Read the model definition and answer for the solid it produces. Units are mm, in the model's axes. A direction names the side the tool comes from. Give positions to 0.01 mm unless a question says otherwise; leave off trailing zeros. Loops run counter-clockwise (first coordinate to the right, second up) from the corner with the lowest first, then second, coordinate; pieces in that order, holes last. Notation, with made-up numbers: (-35, 46) -> (-29, 46) arc R11 cw to (-29, 51) -> close; hole circle Ø9 at (57.25, -1). An arc over 180 degrees is marked (long way). Return JSON: item names as keys, results as strings. Group by question number.
from build123d import *

# Parameters (mm, degrees)
SKETCH1_W           = 195
SKETCH1_H           = 40
BOSS_EXTRUDE1_DEPTH = 10
SKETCH2_W           = 145
SKETCH2_H           = 40
BOSS_EXTRUDE2_DEPTH = 55
CUT_EXTRUDE1_DEPTH  = 237
FILLET1_R           = 7
CUT_EXTRUDE2_DEPTH  = 237
CUT_EXTRUDE3_DEPTH  = 237
SKETCH6_R           = 3
CUT_EXTRUDE4_DEPTH  = 237
SKETCH7_R           = 17.5
BOSS_EXTRUDE3_DEPTH = 2
BOSS_EXTRUDE4_DEPTH = 6
SKETCH9_R           = 4.5
BOSS_EXTRUDE5_DEPTH = 10
BOSS_EXTRUDE7_DEPTH = 5


with BuildPart() as part:
    # Sketch1 → Boss-Extrude1 (new body)
    with BuildSketch(Plane(origin=(0, 0, 0), x_dir=(1, 0, 0), z_dir=(0, 1, 0))):
        Rectangle(SKETCH1_W, SKETCH1_H)
    extrude(amount=BOSS_EXTRUDE1_DEPTH)

    # Sketch2 → Boss-Extrude2 (add)
    with BuildSketch(Plane(origin=(0, 10, 0), x_dir=(1, 0, 0), z_dir=(0, 1, 0))):
        Rectangle(SKETCH2_W, SKETCH2_H)
    extrude(amount=BOSS_EXTRUDE2_DEPTH)

    # Sketch3 → Cut-Extrude1 (cut)
    with BuildSketch(Plane.ZY.offset(72.5)):
        Polygon((-11.5, 65), (-20, 55), (-20, 68.642587118), align=None)
        Polygon((11.5, 65), (20, 55), (20, 68.642587118), align=None)
    extrude(amount=-CUT_EXTRUDE1_DEPTH, mode=Mode.SUBTRACT)

    # Fillet1
    fillet1_edges = [part.edges().sort_by_distance(p)[0] for p in [
        (0, 55, -20),
        (0, 55, 20),
    ]]
    fillet(fillet1_edges, radius=FILLET1_R)

    # Sketch4 → Cut-Extrude2 (cut)
    with BuildSketch(Plane(origin=(0, 0, -20), x_dir=(-1, 0, 0), z_dir=(0, 0, -1))):
        Polygon((72.5, 10), (97.5, 8), (97.5, 10), align=None)
        Polygon((-97.5, 10), (-72.5, 10), (-97.5, 8), align=None)
    extrude(amount=-CUT_EXTRUDE2_DEPTH, mode=Mode.SUBTRACT)

    # Sketch5 → Cut-Extrude3 (cut)
    with BuildSketch(Plane.XZ):
        Polygon((97.5, -20), (97.5, -17.5), (72.5, -20), align=None)
        Polygon((97.5, 20), (72.5, 20), (97.5, 17.5), align=None)
        Polygon((-97.5, 17.5), (-72.5, 20), (-97.5, 20), align=None)
        Polygon((-72.5, -20), (-97.5, -17.5), (-97.5, -20), align=None)
    extrude(amount=-CUT_EXTRUDE3_DEPTH, mode=Mode.SUBTRACT)

    # Sketch6 → Cut-Extrude4 (cut)
    with BuildSketch(Plane.XZ):
        with Locations((89.5, 9)):
            Circle(SKETCH6_R)
        with Locations((89.5, -9)):
            Circle(SKETCH6_R)
        with Locations((-89.5, 9)):
            Circle(SKETCH6_R)
        with Locations((-89.5, -9)):
            Circle(SKETCH6_R)
    extrude(amount=-CUT_EXTRUDE4_DEPTH, mode=Mode.SUBTRACT)

    # Sketch7 → Boss-Extrude3 (add)
    with BuildSketch(Plane(origin=(0, 0, -20), x_dir=(-1, 0, 0), z_dir=(0, 0, -1))):
        with Locations((0, 22.5)):
            Circle(SKETCH7_R)
    extrude(amount=BOSS_EXTRUDE3_DEPTH)

    # Sketch8 → Boss-Extrude4 (add)
    with BuildSketch(Plane(origin=(0, 0, -22), x_dir=(-1, 0, 0), z_dir=(0, 0, -1))):
        Polygon((8.082903769, 8.5), (16.165807537, 22.5), (8.082903769, 36.5), (-8.082903769, 36.5), (-16.165807537, 22.5), (-8.082903769, 8.5), align=None)
    extrude(amount=BOSS_EXTRUDE4_DEPTH)

    # Sketch9 → Boss-Extrude5 (add)
    with BuildSketch(Plane(origin=(0, 0, -28), x_dir=(-1, 0, 0), z_dir=(0, 0, -1))):
        with Locations((0, 22.5)):
            Circle(SKETCH9_R)
    extrude(amount=BOSS_EXTRUDE5_DEPTH)

    # Sketch12 → Boss-Extrude7 (add)
    with BuildSketch(Plane(origin=(0, 0, -38), x_dir=(-1, 0, 0), z_dir=(0, 0, -1))):
        Polygon((2.100473826, 16.281199441), (6.435876178, 21.209663414), (4.335402352, 27.428463972), (-2.100473826, 28.718800559), (-6.435876178, 23.790336586), (-4.335402352, 17.571536028), align=None)
    extrude(amount=BOSS_EXTRUDE7_DEPTH)


solid = part.part
1. Section D-D on y = 34.5 is taken. Determine the outline of the cut face in (x, z), then the cut area to 3 significant figures.
2. Straight lines are drawn through the part: line 1 (X direction, y = 4, z = -9); line 2 (Z direction, x = 89.5, y = 4); line 3 (Z direction, x = -89, y = 3). For each, find the intervals that lie inside material, in ascending order. Write a range as from..to.
3. Section C-C on z = 0 is taken. Determine the outline of the cut face in (x, y).
4. Determine the mould class of faces 1 (the flat face through (72.5, 37, 0)), 2 (the flat face through (-2, 27, -38)), 3 (the cylindrical face through (86.5, 4.4, 9.1)), 4 (the cylindrical face through (-92.5, 4.4, 9.1)) for opening direction X: pulls with the +X half, pulls with the -X half, needs draft (parallel to the pull), parting line crosses it, or undercut.
5. Which of the six approach directions +Z, -Z, +X, -X, +Y, -Y give full straight-line access (tool end or side, diameter ignored) to faces 5 (the flat face through (0, 8, -22)), 6 (the flat face through (4.238, 26.289, -40.465)), 7 (the flat face through (-12.18, 29.4, -24.96)), 8 (the flat face through (-72.5, 37, 0)), 9 (the cylindrical face through (0.59, 26.96, -32.93))?
6. Section A-A on z = 9 is taken. Determine the outline of the cut face in (x, y), then the cut area to 3 significant figures.
7. Flat-ended cylindrical pins translate along their axes: pin 1 Ø6.5 at (x, z) = (3.5, -24) entering from -Y; pin 2 Ø10 at (x, z) = (-60, -17.5) entering from +Y; pin 3 Ø12 at (y, z) = (36, -6.5) entering from +X. Find the tip coordinate at first contact, or state that the pin passes through.
8. Section B-B on x = 89.5 is taken. Determine the outline of the cut face in (y, z), then the cut area to 3 significant figures.
Completed:
{
 "1": {"outline": "(-72.5, -20) -> (-12.74, -20) -> (-12.74, -22) -> (-9.24, -22) -> (-9.24, -28) -> (9.24, -28) -> (9.24, -22) -> (12.74, -22) -> (12.74, -20) -> (72.5, -20) -> (72.5, 20) -> (-72.5, 20) -> close", "area": "5,960 mm²"},
 "2": {"line 1": "x = -97.5..-92.5, -86.5..86.5, 92.5..97.5", "line 2": "z = -18.3..-12, -6..6, 12..18.3", "line 3": "z = -18.35..-11.96, -6.04..6.04, 11.96..18.35"},
 "3": {"outline": "(-97.5, 0) -> (97.5, 0) -> (97.5, 8) -> (72.5, 10) -> (72.5, 65) -> (-72.5, 65) -> (-72.5, 10) -> (-97.5, 8) -> close"},
 "4": {"face 1": "pulls with the +X half", "face 2": "needs draft", "face 3": "undercut", "face 4": "undercut"},
 "5": {"face 5": "-Z", "face 6": "-Z, +X, +Y", "face 7": "-Z, -X, +Y", "face 8": "+Z, -Z, -X, +Y", "face 9": "none"},
 "6": {"outline": "(-97.5, 0) -> (-92.5, 0) -> (-92.5, 8.4) -> (-97.5, 8) -> close; (-86.5, 0) -> (86.5, 0) -> (86.5, 8.88) -> (72.5, 10) -> (72.5, 65) -> (-72.5, 65) -> (-72.5, 10) -> (-86.5, 8.88) -> close; (92.5, 0) -> (97.5, 0) -> (97.5, 8) -> (92.5, 8.4) -> close", "area": "9,770 mm²"},
 "7": {"pin 1": "stops at y = 5.03", "pin 2": "stops at y = 63.82", "pin 3": "stops at x = 72.5"},
 "8": {"outline": "(0, -18.3) -> (8.64, -18.3) -> (8.64, -12) -> (0, -12) -> close; (0, -6) -> (8.64, -6) -> (8.64, 6) -> (0, 6) -> close; (0, 12) -> (8.64, 12) -> (8.64, 18.3) -> (0, 18.3) -> close", "area": "213 mm²"}
}
